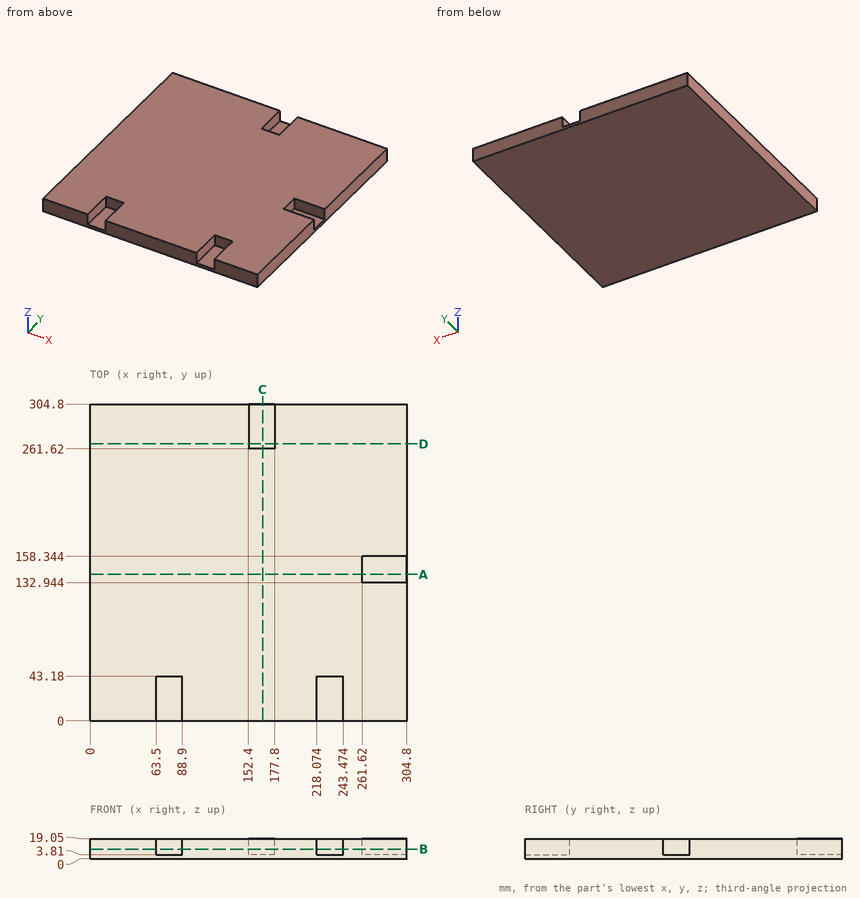
Drawing for the job (mm, zero at the part's lowest x, y, z). Give positions to 0.01 mm unless a question says otherwise; leave off trailing zeros. Write each loop counter-clockwise with the first axis right and the second up, starting at its lowest first coordinate (ties: lowest second). Pieces come first, ordered by that corner, then holes. Notation, with made-up numbers: M -18.75,-31 L 36.25,-31 A37 cw 36.25,6 Z; hole C -26.75,-38.5 d1. An arc over 180 degrees is marked long. Return JSON: item names as keys, results as strings. Group by question number.
(1) Band-saw the part on D-D (y = 266.5). Give the cut face in (x, z), and give its area (3 significant figures).
(2) Band-saw the part on B-B (z = 9.25). Give the cut face in (x, y), and give its area (3 significant figures).
(3) Band-saw the part on A-A (y = 141). Give the cut face in (x, z), and give its area (3 significant figures).
(4) Flat gauge pins, fed straight in: pin 1 Ø12.5 at (x, y) = (234.5, 12) entering from +Z; pin 2 Ø7.5 at (y, z) = (30, 13) entering from -X; pin 3 Ø7.5 at (y, z) = (139.5, 9) entering from +X. Where does each tip first touch, or does it go through?
(5) Drill centre lines: L1, parallel to X at y = 28, z = 5.25; L2, parallel to X at y = 276, z = 8.75; L3, parallel to Y at x = 266, z = 17. Where is each one in solid material? Low to high. Write a range as [from, to].
Entries:
{
 "1": {"outline": "M 0,0 L 304.8,0 L 304.8,19.05 L 177.8,19.05 L 177.8,3.81 L 152.4,3.81 L 152.4,19.05 L 0,19.05 Z", "area": "5,420 mm^2"},
 "2": {"outline": "M 0,0 L 63.5,0 L 63.5,43.18 L 88.9,43.18 L 88.9,0 L 218.07,0 L 218.07,43.18 L 243.47,43.18 L 243.47,0 L 304.8,0 L 304.8,132.94 L 261.62,132.94 L 261.62,158.34 L 304.8,158.34 L 304.8,304.8 L 177.8,304.8 L 177.8,261.62 L 152.4,261.62 L 152.4,304.8 L 0,304.8 Z", "area": "88,500 mm^2"},
 "3": {"outline": "M 0,0 L 304.8,0 L 304.8,3.81 L 261.62,3.81 L 261.62,19.05 L 0,19.05 Z", "area": "5,150 mm^2"},
 "4": {"pin 1": "stops at z = 3.81", "pin 2": "stops at x = 0", "pin 3": "stops at x = 261.62"},
 "5": {"L1": "x = [0, 63.5], [88.9, 218.07], [243.47, 304.8]", "L2": "x = [0, 152.4], [177.8, 304.8]", "L3": "y = [0, 132.94], [158.34, 304.8]"}
}
